The listing builds one solid part. Answer for the finished solid, in the listing's coordinates (mm). A direction names the side the tool comes from. Give positions to 0.01 mm unless a question says otherwise; leave off trailing zeros. Order: outer loops, then holes, each group sorted by start corner. A loop starts at its lowest first (then second) coordinate and runs counter-clockwise, first axis right, second up. Notation, with made-up numbers: (83, 24) -> (128, 24) arc R23 cw to (128, 41) -> close; hole circle Ø11 at (-13.5, -8). An arc over 180 degrees is marked (long way). One line per question, with ' | ' between items. Start each with the question number.
```python
from build123d import *

# Parameters (mm, degrees)
F0_W     = 4.064
F0_H     = 5.08
F1_DEPTH = 12.7
F2_R     = 3.81
F3_DEPTH = 25.4


with BuildPart() as f1:
    # F0 (on Front) → F1 (new body)
    with BuildSketch(Plane.XZ):
        Polygon((-7.62, -8.086451), (0, -8.086451), (7.62, -8.086451), (7.62, 10.963549), (3.556, 10.963549), (2.032, 10.963549), (-2.032, 10.963549), (-3.556, 10.963549), (-7.62, 10.963549), align=None)
        with Locations((0, 13.503549)):
            Rectangle(F0_W, F0_H)
        Polygon((-3.556, 16.043549), (-2.032, 16.043549), (2.032, 16.043549), (3.556, 16.043549), (7.62, 16.043549), (7.62, 41.443549), (0, 41.443549), (-7.62, 41.443549), (-7.62, 16.043549), align=None)
    extrude(amount=F1_DEPTH)

    # F2 (on face) → F3 (cut)
    with BuildSketch(Plane.XZ.offset(12.7)):
        with Locations((0, 31.283549)):
            Circle(F2_R)
    extrude(amount=-F3_DEPTH, mode=Mode.SUBTRACT)


solid = f1.part
```
(1) Consider line 1 (Z direction, x = 0, y = -8.25); line 2 (Z direction, x = 6, y = -6.25); line 3 (Z direction, x = -3.5, y = -6.75). Determine where each line is inside the solid, lowest interval first.
(2) The part is cut by section D-D on x = 0. Determine the outline of the cut face in (y, z).
(3) The part is cut by section C-C on x = -2.75. Determine the outline of the cut face in (y, z).
(4) The part is cut by section A-A on x = 4.5. Determine the outline of the cut face in (y, z).
(5) Determine the mould class of faces 4 (the face through (5, -6, 16.044)), 5 (the face through (7.62, -6, 29)), 6 (the face through (0, -6, 41.444)) for opening direction Z: pulls with the +Z half, pulls with the -Z half, needs draft (parallel to the pull), parting line crosses it, or undercut.
(6) The part is cut by section B-B on y = -6. Determine the outline of the cut face in (x, z).
(7) Given P1, Ø4, axis at y = -8.5, z = 14, coming from the +X side, flat-ended and moving along its own axis, determine where the tip first touches the part or whether it passes through.
(8) For faces 1 (the face through (5, -6, 10.964)), 2 (the face through (0, 0, 17)), 3 (the face through (-5, -6, 16.044)), determine the directions among +Z, -Z, +X, -X, +Y, -Y from which every point of the face is accessible in a straight line to the end or side of a thin tool.
Result sheet:
1) line 1: z = -8.09 to 27.47, 35.09 to 41.44 | line 2: z = -8.09 to 10.96, 16.04 to 41.44 | line 3: z = -8.09 to 10.96, 16.04 to 29.78, 32.79 to 41.44
2) outline: (-12.7, -8.09) -> (0, -8.09) -> (0, 27.47) -> (-12.7, 27.47) -> close; (-12.7, 35.09) -> (0, 35.09) -> (0, 41.44) -> (-12.7, 41.44) -> close
3) outline: (-12.7, -8.09) -> (0, -8.09) -> (0, 10.96) -> (-12.7, 10.96) -> close; (-12.7, 16.04) -> (0, 16.04) -> (0, 28.65) -> (-12.7, 28.65) -> close; (-12.7, 33.92) -> (0, 33.92) -> (0, 41.44) -> (-12.7, 41.44) -> close
4) outline: (-12.7, -8.09) -> (0, -8.09) -> (0, 10.96) -> (-12.7, 10.96) -> close; (-12.7, 16.04) -> (0, 16.04) -> (0, 41.44) -> (-12.7, 41.44) -> close
5) face 4: undercut | face 5: needs draft | face 6: pulls with the +Z half
6) outline: (-7.62, -8.09) -> (7.62, -8.09) -> (7.62, 10.96) -> (2.03, 10.96) -> (2.03, 16.04) -> (7.62, 16.04) -> (7.62, 41.44) -> (-7.62, 41.44) -> (-7.62, 16.04) -> (-2.03, 16.04) -> (-2.03, 10.96) -> (-7.62, 10.96) -> close; hole circle Ø7.62 at (0, 31.28)
7) P1: stops at x = 2.03
8) face 1: +X, +Y, -Y | face 2: +Z, -Z, +X, -X, +Y | face 3: -X, +Y, -Y
